from build123d import *

# Parameters (mm, degrees)
CONTROLLER_REMOVABLE_CENTRAL_TRAY_START   = 57
SKETCH_1_W                                = 70
SKETCH_1_H                                = 134
CONTROLLER_REMOVABLE_CENTRAL_TRAY_DEPTH   = 4
CONTROLLER_FLANGE_AND_SERVICE_SLOTS_START = 62
SKETCH_2_R                                = 1.7
SKETCH_2_W                                = 40
SKETCH_2_H                                = 7
CONTROLLER_FLANGE_AND_SERVICE_SLOTS_DEPTH = 6
DRIVER_POST_AND_FASTENER_CLEARANCE_START  = 62
SKETCH_3_R                                = 4.2
DRIVER_POST_AND_FASTENER_CLEARANCE_DEPTH  = 6


with BuildPart() as part:
    # 草图1 → Controller_removable_central_tray (new body)
    with BuildSketch(Plane.XY.offset(CONTROLLER_REMOVABLE_CENTRAL_TRAY_START)):
        Rectangle(SKETCH_1_W, SKETCH_1_H)
    extrude(amount=CONTROLLER_REMOVABLE_CENTRAL_TRAY_DEPTH)

    # 草图2 → Controller_flange_and_service_slots (cut)
    with BuildSketch(Plane.XY.offset(CONTROLLER_FLANGE_AND_SERVICE_SLOTS_START)):
        with Locations(Location((-30, -62, 0), (0, 0, 180))):
            Circle(SKETCH_2_R)
        with Locations(Location((-30, 62, 0), (0, 0, 180))):
            Circle(SKETCH_2_R)
        with Locations(Location((30, -62, 0), (0, 0, 180))):
            Circle(SKETCH_2_R)
        with Locations(Location((30, 62, 0), (0, 0, 180))):
            Circle(SKETCH_2_R)
        with Locations(Location((15.172281679, -52.5, 0), (0, 0, 180))):
            Circle(SKETCH_2_R)
        with Locations(Location((15.172281679, 52.5, 0), (0, 0, 180))):
            Circle(SKETCH_2_R)
        with Locations(Location((-14.827718321, -52.5, 0), (0, 0, 180))):
            Circle(SKETCH_2_R)
        with Locations(Location((-14.827718321, 52.5, 0), (0, 0, 180))):
            Circle(SKETCH_2_R)
        with Locations((0, -31.5)):
            Rectangle(SKETCH_2_W, SKETCH_2_H)
        with Locations((0, 31.5)):
            Rectangle(SKETCH_2_W, SKETCH_2_H)
    extrude(amount=-CONTROLLER_FLANGE_AND_SERVICE_SLOTS_DEPTH, mode=Mode.SUBTRACT)

    # 草图3 → Driver_post_and_fastener_clearance (cut)
    with BuildSketch(Plane.XY.offset(DRIVER_POST_AND_FASTENER_CLEARANCE_START)):
        with Locations(Location((-22.5, -61, 0), (0, 0, 180))):
            Circle(SKETCH_3_R)
        with Locations(Location((-22.5, 61, 0), (0, 0, 180))):
            Circle(SKETCH_3_R)
        with Locations(Location((22.5, -61, 0), (0, 0, 180))):
            Circle(SKETCH_3_R)
        with Locations(Location((22.5, 61, 0), (0, 0, 180))):
            Circle(SKETCH_3_R)
    extrude(amount=-DRIVER_POST_AND_FASTENER_CLEARANCE_DEPTH, mode=Mode.SUBTRACT)


solid = part.part
Source: CAD feature listing. Evaluate the final solid. Frame: model axes, mm. A direction names the side the tool comes from. Coordinates: 2 decimals unless noted, no trailing zeros. Order: outer loops, then holes, each group sorted by start corner. A loop starts at its lowest first (then second) coordinate and runs counter-clockwise, first axis right, second up. Notation, with made-up numbers: M -2,-10 L 5,-10 A30 cw 5,17 Z; hole C -29,32.5 d5. An arc over 180 degrees is marked long. Write each question's results on one line, items separated by ' | '. Start each with the question number.
Item 1: Cut plane B-B (y = -52.5). Return loops of the section in (x, z).
Item 2: Cut plane A-A (x = -30). Return loops of the section in (y, z).
Item 3: Cut plane C-C (z = 59.8). Count the separate pieces of the cut face and the enclosed holes in it, and give its area (3 significant figures).
Item 4: Draft query along X for faces 3 (the face through (0, 1, 61)), 4 (the face through (35, -1, 59)), 5 (the face through (0, -28, 59)). Return one class per face: pulls with the +X half, pulls with the -X half, needs draft (parallel to the pull), parting line crosses it, or undercut.
Item 5: Line query: probe 1 along X at (y, z) = (-52.5, 58); probe 2 along Y at (x, z) = (-3, 57.9); probe 3 along Y at (x, z) = (-30, 58.95). Output: solid intervals per line, ascending.
Item 6: Set-up query: faces 1 (the face through (0, 67, 59)), 2 (the face through (0, 35, 59)). Return all of +Z, -Z, +X, -X, +Y, -Y with unobstructed straight access to the full face (end or side cutting, diameter ignored); none if empty.
Checked values:
1) outline: M -35,57 L -16.53,57 L -16.53,61 L -35,61 Z; M -13.13,57 L 13.47,57 L 13.47,61 L -13.13,61 Z; M 16.87,57 L 35,57 L 35,61 L 16.87,61 Z
2) outline: M -67,57 L -63.7,57 L -63.7,61 L -67,61 Z; M -60.3,57 L 60.3,57 L 60.3,61 L -60.3,61 Z; M 63.7,57 L 67,57 L 67,61 L 63.7,61 Z
3) separate pieces: 1 | enclosed holes: 14 | area: 8,530 mm2
4) face 3: needs draft | face 4: pulls with the +X half | face 5: undercut
5) probe 1: x = -35 to -16.53, -13.13 to 13.47, 16.87 to 35 | probe 2: y = -67 to -35, -28 to 28, 35 to 67 | probe 3: y = -67 to -63.7, -60.3 to 60.3, 63.7 to 67
6) face 1: +Z, -Z, +X, -X, +Y | face 2: +Z, -Z
